from build123d import *

# Parameters (mm, degrees)
F0_W     = 29
F0_H     = 10
F0_W_2   = 28
F0_H_2   = 9
F1_DEPTH = 10
F2_SIZE  = 0.2


with BuildPart() as f1:
    # F0 (on Front) → F1 (new body)
    with BuildSketch(Plane.XZ):
        with Locations((-8.569464, 10.20826)):
            Rectangle(F0_W, F0_H)
        with Locations((-8.623311, 10.247656)):
            Rectangle(F0_W_2, F0_H_2, mode=Mode.SUBTRACT)
    extrude(amount=F1_DEPTH)

    # F2
    f2_edges = [f1.edges().sort_by_distance(p)[0] for p in [
        (-8.623311, -10, 5.747656),
        (-8.623311, -10, 14.747656),
        (5.376689, -10, 10.247656),
        (-22.623311, -10, 10.247656),
        (-22.623311, 0, 10.247656),
        (-8.623311, 0, 14.747656),
        (-8.623311, 0, 5.747656),
        (5.376689, 0, 10.247656),
    ]]
    chamfer(f2_edges, length=F2_SIZE)


solid = f1.part
For this review, take the finished solid that the model builds, in its own axes (mm). A direction names the side the tool comes from. Give positions to 0.01 mm unless a question says otherwise; leave off trailing zeros. Loops run counter-clockwise (first coordinate to the right, second up) from the corner with the lowest first, then second, coordinate; pieces in that order, holes last. Notation, with made-up numbers: M -12.75,62.25 L 16.25,62.25 A10 ccw 16.25,75.25 Z; hole C 88,-38 d9. An arc over 180 degrees is marked long. Answer as a JSON object with one key per item and string values. Group by question number.
Q1. Add section B-B on x = -13.25. Give the boundary of the cut face in (y, z), and give its area (3 significant figures).
Q2. Mouldability with a two-part tool opening along X and no side actions: class faces 3 (the flat face through (-23.069, -5, 10)), 4 (the flat face through (-9, -5, 15.208)), 5 (the flat face through (-22.623, -5, 10)) as +X half, -X half, draft (parallel to the pull), parting line (faces both ways), or undercut.
Q3. Add section A-A on z = 13.5. Give the boundary of the cut face in (x, y), and give its area (3 significant figures).
Q4. Tool access review of faces 1 (the flat face through (-9, -5, 5.208)), 2 (the flat face through (-9, -5, 5.748)): name each direction out of +Z, -Z, +X, -X, +Y, -Y from which nothing blocks a thin tool from reaching the whole face with its end or side.
Q5. Add section C-C on y = -2.25. Give the boundary of the cut face in (x, z).
Q6. For probe 1 along Z at (x, y) = (-21.5, -8.25); probe 2 along X at (y, z) = (-7.5, 7.5), list the stretches that pass through material, from the lowest coordinate up. Write a range as [from, to].
Checked values:
{
 "1": {"outline": "M -10,5.21 L 0,5.21 L 0,5.55 L -0.2,5.75 L -9.8,5.75 L -10,5.55 Z; M -10,14.95 L -9.8,14.75 L -0.2,14.75 L 0,14.95 L 0,15.21 L -10,15.21 Z", "area": "9.92 mm²"},
 "2": {"face 3": "-X half", "face 4": "draft", "face 5": "undercut"},
 "3": {"outline": "M -23.07,-10 L -22.82,-10 L -22.62,-9.8 L -22.62,-0.2 L -22.82,0 L -23.07,0 Z; M 5.38,-9.8 L 5.58,-10 L 5.93,-10 L 5.93,0 L 5.58,0 L 5.38,-0.2 Z", "area": "9.92 mm²"},
 "4": {"face 1": "-Z, +X, -X, +Y, -Y", "face 2": "+Y, -Y"},
 "5": {"outline": "M -23.07,5.21 L 5.93,5.21 L 5.93,15.21 L -23.07,15.21 Z; hole M -22.62,5.75 L 5.38,5.75 L 5.38,14.75 L -22.62,14.75 Z"},
 "6": {"probe 1": "[5.21, 5.75], [14.75, 15.21]", "probe 2": "[-23.07, -22.62], [5.38, 5.93]"}
}
